from build123d import *

# Parameters (mm, degrees)
F0_W     = 63.346878
F0_H     = 134.601146
F1_DEPTH = 12.7
F2_R     = 5.08
F3_DEPTH = 17.272
F4_W     = 71.3612
F4_H     = 142.089878
F4_W_2   = 29.3665
F4_H_2   = 15.881453
F5_DEPTH = 2.54
F6_R     = 5.08


with BuildPart() as f1:
    # F0 (on Top) → F1 (new body)
    with BuildSketch(Plane.XY):
        with BuildLine():
            Line((29.148949, 71.044939), (-28.998831, 71.044939))
            ThreePointArc((-28.998831, 71.044939), (-33.488959, 69.185067), (-35.348831, 64.694939))
            Line((-35.348831, 64.694939), (-35.348831, -64.845061))
            ThreePointArc((-35.348831, -64.845061), (-33.488959, -69.335189), (-28.998831, -71.195061))
            Line((-28.998831, -71.195061), (29.148949, -71.195061))
            ThreePointArc((29.148949, -71.195061), (33.639077, -69.335189), (35.498949, -64.845061))
            Line((35.498949, -64.845061), (35.498949, 64.694939))
            ThreePointArc((35.498949, 64.694939), (33.639077, 69.185067), (29.148949, 71.044939))
        make_face()
        Rectangle(F0_W, F0_H, mode=Mode.SUBTRACT)
    extrude(amount=F1_DEPTH)

    # F2
    f2_edges = [f1.edges().sort_by_distance(p)[0] for p in [
        (-31.673439, 67.300573, 6.35),
        (31.673439, 67.300573, 6.35),
        (31.673439, -67.300573, 6.35),
        (-31.673439, -67.300573, 6.35),
    ]]
    fillet(f2_edges, radius=F2_R)

    # F0 (on Top) → F3 (join)
    with BuildSketch(Plane.XY):
        with BuildLine():
            Line((29.148949, 71.044939), (-28.998831, 71.044939))
            ThreePointArc((-28.998831, 71.044939), (-33.488959, 69.185067), (-35.348831, 64.694939))
            Line((-35.348831, 64.694939), (-35.348831, -64.845061))
            ThreePointArc((-35.348831, -64.845061), (-33.488959, -69.335189), (-28.998831, -71.195061))
            Line((-28.998831, -71.195061), (29.148949, -71.195061))
            ThreePointArc((29.148949, -71.195061), (33.639077, -69.335189), (35.498949, -64.845061))
            Line((35.498949, -64.845061), (35.498949, 64.694939))
            ThreePointArc((35.498949, 64.694939), (33.639077, 69.185067), (29.148949, 71.044939))
        make_face()
        Rectangle(F0_W, F0_H, mode=Mode.SUBTRACT)
    extrude(amount=F3_DEPTH)

    # F4 (on face) → F5 (join)
    with BuildSketch(Plane.XY.offset(17.272)):
        Rectangle(F4_W, F4_H)
        with Locations((-15.073998, 54.834136)):
            Rectangle(F4_W_2, F4_H_2, mode=Mode.SUBTRACT)
    extrude(amount=F5_DEPTH)

    # F6
    f6_edges = [f1.edges().sort_by_distance(p)[0] for p in [
        (-35.6806, 71.044939, 18.542),
        (35.6806, 71.044939, 18.542),
        (35.6806, -71.044939, 18.542),
        (-35.6806, -71.044939, 18.542),
    ]]
    fillet(f6_edges, radius=F6_R)


solid = f1.part
Build history of the part. All positions in model axes, mm. A direction names the side the tool comes from. Give positions to 0.01 mm unless a question says otherwise; leave off trailing zeros. Order: outer loops, then holes, each group sorted by start corner. A loop starts at its lowest first (then second) coordinate and runs counter-clockwise, first axis right, second up. Notation, with made-up numbers: M 27,62.5 L 31,62.5 A10 cw 31,72.5 Z; hole C 83.25,33 d7. An arc over 180 degrees is marked long. Put each result on its own line as item: value.
Item 1: 3-axis set-ups, long thin cutter, end or side, ignore diameter. For faces 4 (the cylindrical face through (33.589, -69.384, 8.515)), 5 (the cylindrical face through (-33.538, -69.286, 8.515)), 6 (the flat face through (-31, 66, 12.7)), 7 (the flat face through (-29.757, 55, 19)), 8 (the flat face through (0, -71.045, 19)): which of +Z, -Z, +X, -X, +Y, -Y reach the whole face in a straight line?
From the geometry:
face 4: -Z, +X, -Y
face 5: -Z, -X, -Y
face 6: none
face 7: +Z, -Z
face 8: +Z, +X, -X, -Y
Item 2: Slice it at D-D, the plane x = 6.5. Write the cut outline in (y, z).
From the geometry:
outline: M -71.2,0 L -67.3,0 L -67.3,17.27 L 67.3,17.27 L 67.3,0 L 71.04,0 L 71.04,19.81 L -71.04,19.81 L -71.04,17.27 L -71.2,17.27 Z
Item 3: Slice it at B-B, the plane y = 51.5. Write the cut outline in (x, z), plus the area to 3 significant figures.
From the geometry:
outline: M -35.68,17.27 L -35.35,17.27 L -35.35,0 L -31.67,0 L -31.67,17.27 L -29.76,17.27 L -29.76,19.81 L -35.68,19.81 Z; M -0.39,17.27 L 31.67,17.27 L 31.67,0 L 35.5,0 L 35.5,17.27 L 35.68,17.27 L 35.68,19.81 L -0.39,19.81 Z
area: 236 mm2
Item 4: Two-plate mould, pull along X, no slides. Class faces 1 (the flat face through (-34, 0, 0)), 2 (the flat face through (-31, -66, 12.7)), 3 (the cylindrical face through (-33.439, 69.234, 8.515)): +X half, -X half, draft (parallel to the pull), parting line (faces both ways), or undercut.
From the geometry:
face 1: draft
face 2: undercut
face 3: -X half
Item 5: Slice it at C-C, the plane z = 5.75. Write the cut outline in (x, y), plus the area to 3 significant figures.
From the geometry:
outline: M -35.35,-64.85 A6.35 ccw -29,-71.2 L 29.15,-71.2 A6.35 ccw 35.5,-64.85 L 35.5,64.69 A6.35 ccw 29.15,71.04 L -29,71.04 A6.35 ccw -35.35,64.69 Z; hole M -31.67,-62.22 A5.08 ccw -26.59,-67.3 L 26.59,-67.3 A5.08 ccw 31.67,-62.22 L 31.67,62.22 A5.08 ccw 26.59,67.3 L -26.59,67.3 A5.08 ccw -31.67,62.22 Z
area: 1,540 mm2
Item 6: Probe line 1 (X direction, y = -36, z = 16); line 2 (Y direction, x = -12.5, z = 13); line 3 (Z direction, x = -15.5, y = -60.5). List the from-to ranges inside material, lowest first. Write a range as [from, to].
From the geometry:
line 1: x = [-35.35, -31.67], [31.67, 35.5]
line 2: y = [-71.2, -67.3], [67.3, 71.04]
line 3: z = [17.27, 19.81]
Item 7: Flat gauge pins, fed straight in: pin 1 Ø1 at (y, z) = (-7, 6) entering from -X; pin 2 Ø1.3 at (x, z) = (-5, 19) entering from -Y; pin 3 Ø3 at (x, y) = (-22, 11.5) entering from -Z. Where does each tip first touch, or does it go through?
From the geometry:
pin 1: stops at x = -35.35
pin 2: stops at y = -71.04
pin 3: stops at z = 17.27
Item 8: Slice it at A-A, the plane x = -25. Write the cut outline in (y, z), plus the area to 3 significant figures.
From the geometry:
outline: M -71.2,0 L -67.3,0 L -67.3,17.27 L 46.89,17.27 L 46.89,19.81 L -71.04,19.81 L -71.04,17.27 L -71.2,17.27 Z; M 62.77,17.27 L 67.3,17.27 L 67.3,0 L 71.04,0 L 71.04,19.81 L 62.77,19.81 Z
area: 453 mm2
